from build123d import *

# Parameters (mm, degrees)
CROQUIS1_W              = 34
CROQUIS1_H              = 15
CROQUIS1_W_2            = 10
CROQUIS1_H_2            = 10
SALIENTE_EXTRUIR1_DEPTH = 5


with BuildPart() as part:
    # Croquis1 → Saliente-Extruir1 (new body)
    # profile 1 of 2: a face of its own
    with BuildSketch(Plane.XY):
        Rectangle(CROQUIS1_W, CROQUIS1_H)
        Rectangle(CROQUIS1_W_2, CROQUIS1_H_2, mode=Mode.SUBTRACT)
    # profile 2 of 2: a face of its own
    with BuildSketch(Plane.XY):
        Polygon((17, -7.5), (7.100505063, -17.399494937), (7.100505063, -37.399494937), (-7.100505063, -37.399494937), (-7.100505063, -17.399494937), (-17, -7.5), align=None)
    extrude(amount=SALIENTE_EXTRUIR1_DEPTH)


solid = part.part
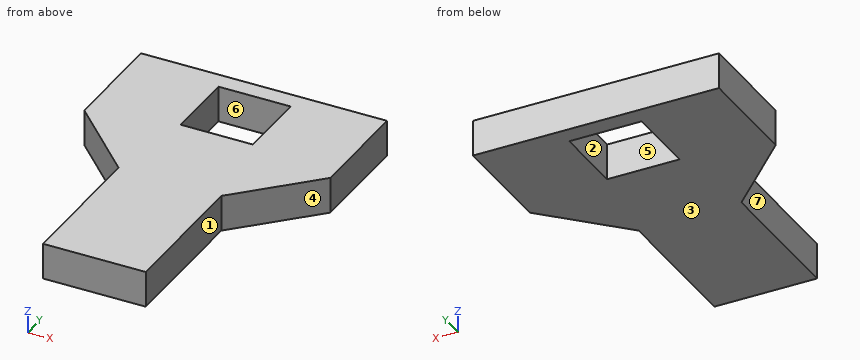
Could you check a few things on this model? Use its own coordinates, in mm. Face numbers are marked on the shaded views. A direction names the side the tool comes from. Round coordinates to 2 decimals unless told otherwise and drop trailing zeros. Order: outer loops, then holes, each group sorted by start corner. A loop starts at its lowest first (then second) coordinate and runs counter-clockwise, first axis right, second up.
(1) Which directions (+Z, -Z, +X, -X, +Y, -Y) give clear straight access to the entire face, cutting with the end or side of a thin tool? Please do the marked faces 1, 2 and 3.
Response values:
face 1: +Z, -Z, +X, -Y
face 2: +Z, -Z
face 3: -Z, +X, -X, +Y, -Y
(2) I'm going to push flat-ended pins straight in: pin 1 (1 mm diameter, centred on x = 9, y = -12, fed in from -Z); pin 2 (1 mm diameter, centred on x = 10, z = 2.5, fed in from -Y); pin 3 (3 mm diameter, centred on x = -9.5, z = 4.5, fed in from -Y). Where does each tip first touch, or does it pass through?
Response values:
pin 1: stops at z = 0
pin 2: stops at y = -15
pin 3: stops at y = -16.5
(3) Imagine slicing it at B-B (y = -2.5). Write out the boundary of the cut face in (x, z).
Response values:
outline: (-17, 0) - (-5, 0) - (-5, 5) - (-17, 5) - close; (5, 0) - (17, 0) - (17, 5) - (5, 5) - close
(4) Please list where these lines run through material, in increasing order: line 1 along Y through (x, z) = (-2.5, 4.3); line 2 along X through (y, z) = (-3.5, 2.1); line 3 along X through (y, z) = (-31.5, 3.35).
Response values:
line 1: y = -37.4 to -5, 5 to 7.5
line 2: x = -17 to -5, 5 to 17
line 3: x = -7.1 to 7.1
(5) Imagine slicing it at D-D (y = -31). Write out the boundary of the cut face in (x, z), plus the area to 3 significant figures.
Response values:
outline: (-7.1, 0) - (7.1, 0) - (7.1, 5) - (-7.1, 5) - close
area: 71.0 mm2
(6) Imagine slicing it at C-C (z = 2.75). Write out the boundary of the cut face in (x, y), plus the area to 3 significant figures.
Response values:
outline: (-17, -7.5) - (-7.1, -17.4) - (-7.1, -37.4) - (7.1, -37.4) - (7.1, -17.4) - (17, -7.5) - (17, 7.5) - (-17, 7.5) - close; hole (-5, -5) - (5, -5) - (5, 5) - (-5, 5) - close
area: 933 mm2
(7) If we mould it in two halves opening along Y, with no side actions, what happens to the marked faces 4, 5, 6 and 7? For each: released by +Y, released by -Y, zero draft, split by the parting line, or undercut.
Response values:
face 4: released by -Y
face 5: undercut
face 6: undercut
face 7: zero draft
(8) Imagine slicing it at A-A (x = 3). Write out the boundary of the cut face in (y, z), plus the area to 3 significant figures.
Response values:
outline: (-37.4, 0) - (-5, 0) - (-5, 5) - (-37.4, 5) - close; (5, 0) - (7.5, 0) - (7.5, 5) - (5, 5) - close
area: 174 mm2
